Part model, mm, in its own coordinate system. A direction names the side the tool comes from. Coordinates: 2 decimals unless noted, no trailing zeros. Loops run counter-clockwise (first coordinate to the right, second up) from the corner with the lowest first, then second, coordinate; pieces in that order, holes last. Notation, with made-up numbers: (56, 80.5) - (102, 80.5) arc R14 ccw to (102, 107.5) - close; hole circle Ø3 at (68, 23.25). An arc over 180 degrees is marked (long way). Use a Markdown table: item, result. Add a question column.
1. Band-saw the part on C-C, the plane z = 0. Count the separate pieces of the cut face and the enclosed holes in it, plus the area to 3 significant figures.
2. Wall check: probe 1 along Y at (x, z) = (0.65, 0); probe 2 along Y at (x, z) = (42, 0). Give the ranges that are in metal, low to high. Write a range as [from, to].
3. Drop flat-ended pins along their axis: pin 1 (1 mm diameter, centred on x = 47.5, y = 1, fed in from -Z); pin 2 (4.5 mm diameter, centred on x = 31.75, z = 0, fed in from +Y); pin 3 (12.5 mm diameter, centred on y = 9.5, z = 5, fed in from +X). Give the stop position or say it passes through.
4. Band-saw the part on B-B, the plane z = -3. Give the cut face in (x, y), plus the area to 3 significant figures.
5. 3-axis set-ups, long thin cutter, end or side, ignore diameter. For faces 1 (the cylindrical face through (7.61, 1, 12)), 2 (the cylindrical face through (7.585, 1.002, -12.021)), 3 (the cylindrical face through (42.8, 1.03, -0.07)), 4 (the flat face through (2.032, 13, -3)): which of +Z, -Z, +X, -X, +Y, -Y reach the whole face in a straight line?
6. Pull direction X, two halves, no side cores. Call faces 5 (the flat face through (0, 13, -3)), 6 (the cylindrical face through (31.913, 1.002, 12.446)), 7 (the cylindrical face through (51.572, 1.03, -11.974)), 8 (the cylindrical face through (1, 9.39, 0.89)): pulls with the +X half, pulls with the -X half, needs draft (parallel to the pull), parting line crosses it, or undercut.
7. Band-saw the part on A-A, the plane x = 19.05. Give the cut face in (y, z), plus the area to 3 significant figures.
8. Band-saw the part on D-D, the plane y = 22. Give the cut face in (x, z), plus the area to 3 significant figures.
from build123d import *

# Parameters (mm, degrees)
BOSS_EXTRUDE1_DEPTH      = 2.032
SKETCH2_W                = 24.892
SKETCH2_H                = 2.032
BOSS_EXTRUDE2_DEPTH      = 7.366000072
SKETCH3_W                = 24.892
SKETCH3_H                = 2.032
BOSS_EXTRUDE3_DEPTH      = 4.318000079
BOSS_EXTRUDE4_DEPTH      = 2.032
M7_CLEARANCE_HOLE1_D     = 7.62
M3_CLEARANCE_HOLE1_D     = 3.302
M3_CLEARANCE_HOLE2_D     = 3.302
M3_CLEARANCE_HOLE2_DEPTH = 28.956
FILLET1_R                = 1.655535703
FILLET2_R                = 2.032


with BuildPart() as part:
    # Sketch1 → Boss-Extrude1 (new body)
    with BuildSketch(Plane.XZ):
        with BuildLine():
            Line((44.703999934, -12.446), (44.703999934, 12.446))
            ThreePointArc((44.703999934, 12.446), (43.455024595, 12.008165774), (42.926000003, 10.795000003))
            ThreePointArc((42.926000003, 10.795000003), (41.402000003, 9.271000003), (39.878000003, 10.795000003))
            ThreePointArc((39.878000003, 10.795000003), (38.227000003, 12.446000003), (36.576000003, 10.795000003))
            ThreePointArc((36.576000003, 10.795000003), (35.052000003, 9.271000003), (33.528000003, 10.795000003))
            ThreePointArc((33.528000003, 10.795000003), (31.877000003, 12.446000003), (30.226000003, 10.795000003))
            ThreePointArc((30.226000003, 10.795000003), (28.702000003, 9.271000003), (27.178000003, 10.795000003))
            ThreePointArc((27.178000003, 10.795000003), (25.527000003, 12.446000003), (23.876000003, 10.795000003))
            ThreePointArc((23.876000003, 10.795000003), (22.352000003, 9.271000003), (20.828000003, 10.795000003))
            ThreePointArc((20.828000003, 10.795000003), (19.177000003, 12.446000003), (17.526000003, 10.795000003))
            ThreePointArc((17.526000003, 10.795000003), (16.002000003, 9.271000003), (14.478000003, 10.795000003))
            ThreePointArc((14.478000003, 10.795000003), (12.827000003, 12.446000003), (11.176000003, 10.795000003))
            ThreePointArc((11.176000003, 10.795000003), (9.652000003, 9.271000003), (8.128000003, 10.795000003))
            ThreePointArc((8.128000003, 10.795000003), (7.598975413, 12.008165771), (6.350000079, 12.446))
            Line((6.350000079, 12.446), (6.350000079, -12.446))
            ThreePointArc((6.350000079, -12.446), (7.598975413, -12.008165771), (8.128000003, -10.795000003))
            ThreePointArc((8.128000003, -10.795000003), (9.652000003, -9.271000003), (11.176000003, -10.795000003))
            ThreePointArc((11.176000003, -10.795000003), (12.827000003, -12.446000003), (14.478000003, -10.795000003))
            ThreePointArc((14.478000003, -10.795000003), (16.002000003, -9.271000003), (17.526000003, -10.795000003))
            ThreePointArc((17.526000003, -10.795000003), (19.177000003, -12.446000003), (20.828000003, -10.795000003))
            ThreePointArc((20.828000003, -10.795000003), (22.352000003, -9.271000003), (23.876000003, -10.795000003))
            ThreePointArc((23.876000003, -10.795000003), (25.527000003, -12.446000003), (27.178000003, -10.795000003))
            ThreePointArc((27.178000003, -10.795000003), (28.702000003, -9.271000003), (30.226000003, -10.795000003))
            ThreePointArc((30.226000003, -10.795000003), (31.877000003, -12.446000003), (33.528000003, -10.795000003))
            ThreePointArc((33.528000003, -10.795000003), (35.052000003, -9.271000003), (36.576000003, -10.795000003))
            ThreePointArc((36.576000003, -10.795000003), (38.227000003, -12.446000003), (39.878000003, -10.795000003))
            ThreePointArc((39.878000003, -10.795000003), (41.402000003, -9.271000003), (42.926000003, -10.795000003))
            ThreePointArc((42.926000003, -10.795000003), (43.455024595, -12.008165773), (44.703999934, -12.446))
        make_face()
    extrude(amount=-BOSS_EXTRUDE1_DEPTH)

    # Sketch2 → Boss-Extrude2 (add)
    with BuildSketch(Plane(origin=(44.703999934, 0, 0), x_dir=(0, 0, -1), z_dir=(1, 0, 0))):
        with Locations((0, 1.016)):
            Rectangle(SKETCH2_W, SKETCH2_H)
    extrude(amount=BOSS_EXTRUDE2_DEPTH)

    # Sketch3 → Boss-Extrude3 (add)
    with BuildSketch(Plane.ZY.offset(-6.350000079)):
        with Locations((0, 1.016)):
            Rectangle(SKETCH3_W, SKETCH3_H)
    extrude(amount=BOSS_EXTRUDE3_DEPTH)

    # Sketch4 → Boss-Extrude4 (add)
    with BuildSketch(Plane.ZY.offset(-2.032)):
        with BuildLine():
            Line((-12.446, 0), (-12.446, 16.51))
            ThreePointArc((-12.446, 16.51), (0, 28.956), (12.446, 16.51))
            Line((12.446, 16.51), (12.446, 0))
            Line((12.446, 0), (-12.446, 0))
        make_face()
    extrude(amount=BOSS_EXTRUDE4_DEPTH)

    # M7 Clearance Hole1 (through all)
    with Locations(Plane(origin=(2.032, 0, 0), x_dir=(0, 0, -1), z_dir=(1, 0, 0))):
        with Locations((0, 16.51)):
            Hole(M7_CLEARANCE_HOLE1_D / 2)

    # M3 Clearance Hole1 (through all)
    with Locations(Plane(origin=(2.032, 0, 0), x_dir=(0, 0, -1), z_dir=(1, 0, 0))):
        with Locations((0, 25.019), (0, 8.001), (-8.509, 16.51), (8.509, 16.51)):
            Hole(M3_CLEARANCE_HOLE1_D / 2)

    # M3 Clearance Hole2
    with Locations(Plane(origin=(0, 0, 0), x_dir=(-1, 0, 0), z_dir=(0, -1, 0))):
        with Locations((-38.1, 0), (-25.4, 0), (-12.7, 0), (-6.35, 0), (-19.05, 0), (-31.75, 0), (-44.45, 0)):
            Hole(M3_CLEARANCE_HOLE2_D / 2, depth=M3_CLEARANCE_HOLE2_DEPTH)

    # Fillet1
    fillet1_edges = [part.edges().sort_by_distance(p)[0] for p in [
        (52.070000006, 1.016, -12.446),
        (52.070000006, 1.016, 12.446),
    ]]
    fillet(fillet1_edges, radius=FILLET1_R)

    # Fillet2
    fillet2_edges = [part.edges().sort_by_distance(p)[0] for p in [
        (0, 0, 0),
    ]]
    fillet(fillet2_edges, radius=FILLET2_R)


solid = part.part
Geometry check:
| question | item | result |
|---|---|---|
| 1 | separate pieces | 11 |
| 1 | enclosed holes | 0 |
| 1 | area | 83.8 mm^2 |
| 2 | probe 1 | y = [0.54, 6.35], [9.65, 12.7], [20.32, 23.37], [26.67, 28.96] |
| 2 | probe 2 | y = [0, 2.03] |
| 3 | pin 1 | stops at z = -12.45 |
| 3 | pin 2 | stops at y = 2.03 |
| 3 | pin 3 | stops at x = 2.03 |
| 4 | outline | (0, 2.03) arc R2.03 ccw to (2.03, 0) - (52.07, 0) - (52.07, 2.03) - (2.03, 2.03) - (2.03, 14.16) - (0, 14.16) - close; (0, 18.86) - (2.03, 18.86) - (2.03, 28.59) - (0, 28.59) - close |
| 4 | area | 149 mm^2 |
| 5 | face 1 | +Z, +Y, -Y |
| 5 | face 2 | -Z, +Y, -Y |
| 5 | face 3 | +Y, -Y |
| 5 | face 4 | +Z, -Z, +X, +Y |
| 6 | face 5 | pulls with the -X half |
| 6 | face 6 | undercut |
| 6 | face 7 | pulls with the +X half |
| 6 | face 8 | needs draft |
| 7 | outline | (0, -12.44) - (2.03, -12.44) - (2.03, -1.65) - (0, -1.65) - close; (0, 1.65) - (2.03, 1.65) - (2.03, 12.44) - (0, 12.44) - close |
| 7 | area | 43.9 mm^2 |
| 8 | outline | (0, -11.17) - (2.03, -11.17) - (2.03, 11.17) - (0, 11.17) - close |
| 8 | area | 45.4 mm^2 |
